Geometry: final body of the model. Coordinates: model frame, mm. A direction names the side the tool comes from. Round coordinates to 2 decimals unless told otherwise and drop trailing zeros. Order: outer loops, then holes, each group sorted by start corner. A loop starts at its lowest first (then second) coordinate and runs counter-clockwise, first axis right, second up. Notation, with made-up numbers: (-12, 38) - (5, 38) arc R27 cw to (5, 59) - close; hole circle Ø5 at (-13, -2). An arc over 180 degrees is marked (long way). Put each result on its own line as item: value. Start each with the question number.
(1) Material intervals for L1, parallel to Y at x = 14.6, z = 2; L2, parallel to X at y = 1.5, z = 5.5; L3, parallel to X at y = 3, z = 4, sorted ascending. Write a range as [from, to].
(2) Section B-B (x = 14.6). Output: boundary loops of the cut face in (y, z).
(3) Section D-D (z = 3.2). Count the separate pieces of the cut face and the enclosed holes in it, and give its area (3 significant figures).
(4) Access query for faces 1 (the face through (1.6, -1.5, 3.5)), 2 (the face through (8.9, -1.5, 3.5)), 3 (the face through (8.6, 10.2, 3.2)), 4 (the face through (18.2, -1.5, 2.9)), 5 (the face through (3, 10.2, 3)). Directions: +Z, -Z, +X, -X, +Y, -Y. A direction counts if a zero-diameter tool reaches every point of the face in a straight line with its end or side. Return the directions, or none.
(5) Pull-direction query (X, two-part tool) for faces 6 (the face through (10, 5, 6.4)), 7 (the face through (19.8, 4, 3)), 8 (the face through (2.1, -1.5, 2.9)); classes: released by +X, released by -X, zero draft, split by the parting line, or undercut.
(6) Section C-C (z = 4.5). Output: boundary loops of the cut face in (x, y), and give its area (3 significant figures).
(7) Section A-A (y = 2.5). Output: boundary loops of the cut face in (x, z).
(8) Pin query (flat end, axial travel): P1, Ø2, axis at x = 11.5, z = 5.5, coming from the +Y side; P2, Ø0.6, axis at x = 9, y = -1.5, coming from the +Z side; P3, Ø3.5, axis at y = -2, z = 2.5, coming from the +X side. Return the tip coordinate at first contact, or that it passes through.
Autodesk Inventor part; units mm, degrees
ref_plane "YZ Plane" through (0, 0, 0) normal (1, 0, 0) x (0, 1, 0)
ref_plane "XZ Plane" through (0, 0, 0) normal (0, 1, 0) x (-1, 0, 0)
ref_plane "XY Plane" through (0, 0, 0) normal (0, 0, 1) x (1, 0, 0)
sketch "Sketch1" plane through (0, 0, 0) normal (0, 0, 1) x (1, 0, 0)
  line L0 (0, 0) -> (0, 10.2)
  line L1 (0, 10.2) -> (9.1, 10.2)
  line L2 (9.1, 10.2) -> (9.99, 8.6487)
  line L3 (9.99, 8.6487) -> (19.8, 8.6487)
  line L4 (19.8, 8.6487) -> (19.8, 0)
  line L5 (19.8, 0) -> (0, 0)
  circle A0 centre (5.1, 2.5) radius 1.25
  circle A1 centre (14.6, 2.5) radius 1.25
  arc A2 (8.1, 10.5) -> (6.1001, 10.4874) centre (7.1, 10.5) ccw
  line L6 (8.1, 10.5) -> (8.1, 10.2)
  line L7 (6.1001, 10.5) -> (6.1001, 10.2)
  dimension "d0" = 9.1
  dimension "d1" = 10.2
  dimension "d2" = 19.8
  dimension "d3" = 2.5
  dimension "d4" = 5.1
  dimension "d5" = 2.5
  dimension "d6" = 9.5
  dimension "d7" = 2.5
  dimension "d8" = 2.5
  dimension "d9" = 2
  dimension "d10" = 7.5
  dimension "d11" = 10.5
extrude "Extrusion1" add sketch "Sketch1" along normal blind 6.4
sketch "Sketch3" plane through (0, 0, 0) normal (0, -1, 0) x (1, 0, 0)
  line L0 (8.9, 1.6) -> (8.9, 4.8)
  line L1 (8.9, 4.8) -> (9.4, 4.8)
  line L2 (9.4, 4.8) -> (9.4, 1.6)
  line L3 (9.4, 1.6) -> (8.9, 1.6)
  line L4 (17.7, 1.6) -> (17.7, 4.8)
  line L5 (17.7, 4.8) -> (18.2, 4.8)
  line L6 (18.2, 4.8) -> (18.2, 1.6)
  line L7 (18.2, 1.6) -> (17.7, 1.6)
  line L8 (1.6, 1.6) -> (1.6, 4.8)
  line L9 (1.6, 4.8) -> (2.1, 4.8)
  line L10 (2.1, 4.8) -> (2.1, 1.6)
  line L11 (2.1, 1.6) -> (1.6, 1.6)
extrude "Extrusion3" add sketch "Sketch3" along normal blind 4
sketch "Sketch4" plane through (18.2, 0, 4.8) normal (1, 0, 0) x (0, 0, -1)
  circle A0 centre (1.6, -2.4215) radius 0.8
  point P0 (4.8, 0)
  dimension "d24" = 1.6
extrude "Extrusion4" cut sketch "Sketch4" against normal blind 22
sketch "Sketch2" plane through (0, 0, 6.4) normal (0, 0, 1) x (1, 0, 0)
  line L0 (1.6916, 0) -> (2.1916, 0)
  line L1 (2.1916, 0) -> (2.1916, -4)
  line L2 (2.1916, -4) -> (1.6916, -4)
  line L3 (1.6916, -4) -> (1.6916, 0)
  line L4 (10.4916, 0) -> (10.9916, 0)
  line L5 (10.9916, 0) -> (10.9916, -4)
  line L6 (10.9916, -4) -> (10.4916, -4)
  line L7 (10.4916, -4) -> (10.4916, 0)
  line L8 (17.7916, 0) -> (18.2916, 0)
  line L9 (18.2916, 0) -> (18.2916, -4)
  line L10 (18.2916, -4) -> (17.7916, -4)
  line L11 (17.7916, -4) -> (17.7916, 0)
  point P0 (0, 0)
  point P1 (-19.8, 0)
  dimension "d14" = 0.5
  dimension "d15" = 4
  dimension "d16" = 0.5
  dimension "d17" = 0.5
  dimension "d18" = 8.3
  dimension "d19" = 6.8
properties part number "endstop"
Checks:
1. L1: y = [0, 1.25], [3.75, 8.65]
1. L2: x = [0, 4.35], [5.85, 13.85], [15.35, 19.8]
1. L3: x = [0, 3.95], [6.25, 13.45], [15.75, 19.8]
2. outline: (0, 0) - (1.25, 0) - (1.25, 6.4) - (0, 6.4) - close; (3.75, 0) - (8.65, 0) - (8.65, 6.4) - (3.75, 6.4) - close
3. separate pieces: 4
3. enclosed holes: 2
3. area: 182 mm²
4. face 1: +Z, -Z, -X, -Y
4. face 2: +Z, -Z, -Y
4. face 3: +Z, -Z, +X, +Y
4. face 4: +Z, -Z, +X, -Y
4. face 5: +Z, -Z, -X, +Y
5. face 6: zero draft
5. face 7: released by +X
5. face 8: undercut
6. outline: (0, 0) - (1.6, 0) - (1.6, -4) - (2.1, -4) - (2.1, 0) - (8.9, 0) - (8.9, -4) - (9.4, -4) - (9.4, 0) - (17.7, 0) - (17.7, -4) - (18.2, -4) - (18.2, 0) - (19.8, 0) - (19.8, 8.65) - (9.99, 8.65) - (9.1, 10.2) - (8.1, 10.2) - (8.1, 10.5) arc R1 ccw (long way) to (6.1, 10.49) - (6.1, 10.2) - (0, 10.2) - close; hole circle Ø2.5 at (5.1, 2.5); hole circle Ø2.5 at (14.6, 2.5)
6. area: 184 mm²
7. outline: (0, 0) - (3.85, 0) - (3.85, 6.4) - (0, 6.4) - close; (6.35, 0) - (13.35, 0) - (13.35, 6.4) - (6.35, 6.4) - close; (15.85, 0) - (19.8, 0) - (19.8, 6.4) - (15.85, 6.4) - close
8. P1: stops at y = 8.65
8. P2: stops at z = 4.8
8. P3: stops at x = 18.2
